from build123d import *

# Parameters (mm, degrees)
SKETCH_1_W                       = 990
SKETCH_1_H                       = 2
SM_BASE_FLANGE_1_DEPTH           = 60
SM_EDGE_FLANGE_1_STRIP_W         = 9
SM_EDGE_FLANGE_1_STRIP_H         = 2
SM_EDGE_FLANGE_1_STRIP_CUT_DEPTH = 990
SM_EDGE_FLANGE_1_DEPTH           = 990
SM_EDGE_FLANGE_2_STRIP_W         = 9
SM_EDGE_FLANGE_2_STRIP_H         = 2
SM_EDGE_FLANGE_2_STRIP_CUT_DEPTH = 990
SM_EDGE_FLANGE_2_DEPTH           = 990
SM_EDGE_FLANGE_3_STRIP_W         = 9
SM_EDGE_FLANGE_3_STRIP_H         = 2
SM_EDGE_FLANGE_3_STRIP_CUT_DEPTH = 990
SM_EDGE_FLANGE_3_DEPTH           = 990
SM_EDGE_FLANGE_4_STRIP_W         = 9
SM_EDGE_FLANGE_4_STRIP_H         = 2
SM_EDGE_FLANGE_4_STRIP_CUT_DEPTH = 990
SM_EDGE_FLANGE_4_DEPTH           = 990
HOLE_WIZARD_19_0_19_1_D          = 19
HOLE_WIZARD_M4_1_D               = 4
PATTERN_LINEAR_1_COUNT           = 2
PATTERN_LINEAR_1_PITCH           = 764.04
CUT_EXTRUDE_1_DEPTH              = 2
PATTERN_LINEAR_2_COUNT           = 2
PATTERN_LINEAR_2_PITCH           = 20
PATTERN_LINEAR_2_COUNT_DIR2      = 2
PATTERN_LINEAR_2_PITCH_DIR2      = 35
CUT_EXTRUDE_4_DEPTH              = 2
MIRROR_1_COPY_1_DEPTH            = 2
MIRROR_1_COPY_2_DEPTH            = 2
MIRROR_1_COPY_3_DEPTH            = 2
CUT_EXTRUDE_2_DEPTH              = 2
PATTERN_LINEAR_3_COUNT           = 6
PATTERN_LINEAR_3_PITCH           = 116


# Sheet-metal steps are written as plain solids
with BuildPart() as part:
    # Sketch 1 → 基体-法兰1 (new body)
    with BuildSketch(Plane.XY):
        with Locations((0, -1)):
            Rectangle(SKETCH_1_W, SKETCH_1_H)
    extrude(amount=SM_BASE_FLANGE_1_DEPTH)

    # 边线-法兰1 strip (across the edge) → 边线-法兰1 strip cut (cut)
    with BuildSketch(Plane(origin=(-495, -2, 0), x_dir=(0, 0, 1), z_dir=(1, 0, 0))):
        with Locations((-2, -1)):
            Rectangle(SM_EDGE_FLANGE_1_STRIP_W, SM_EDGE_FLANGE_1_STRIP_H)
    extrude(amount=SM_EDGE_FLANGE_1_STRIP_CUT_DEPTH, mode=Mode.SUBTRACT)

    # 边线-法兰1 section (across the edge) → 边线-法兰1 (add)
    with BuildSketch(Plane(origin=(-495, -2, 0), x_dir=(0, 0, 1), z_dir=(1, 0, 0))):
        with BuildLine():
            Line((0, 0.5), (0, 15))
            Line((0, 15), (2, 15))
            Line((2, 15), (2, 0.5))
            ThreePointArc((2, 0.5), (2.146446609, 0.146446609), (2.5, 0))
            Line((2.5, 0), (2.5, -2))
            ThreePointArc((2.5, -2), (0.732233047, -1.267766953), (0, 0.5))
        make_face()
    extrude(amount=SM_EDGE_FLANGE_1_DEPTH)

    # 边线-法兰2 strip (across the edge) → 边线-法兰2 strip cut (cut)
    with BuildSketch(Plane(origin=(495, -2, 60), x_dir=(0, 0, -1), z_dir=(-1, 0, 0))):
        with Locations((-2, -1)):
            Rectangle(SM_EDGE_FLANGE_2_STRIP_W, SM_EDGE_FLANGE_2_STRIP_H)
    extrude(amount=SM_EDGE_FLANGE_2_STRIP_CUT_DEPTH, mode=Mode.SUBTRACT)

    # 边线-法兰2 section (across the edge) → 边线-法兰2 (add)
    with BuildSketch(Plane(origin=(495, -2, 60), x_dir=(0, 0, -1), z_dir=(-1, 0, 0))):
        with BuildLine():
            Line((0, 0.5), (0, 15))
            Line((0, 15), (2, 15))
            Line((2, 15), (2, 0.5))
            ThreePointArc((2, 0.5), (2.146446609, 0.146446609), (2.5, 0))
            Line((2.5, 0), (2.5, -2))
            ThreePointArc((2.5, -2), (0.732233047, -1.267766953), (0, 0.5))
        make_face()
    extrude(amount=SM_EDGE_FLANGE_2_DEPTH)

    # 边线-法兰3 strip (across the edge) → 边线-法兰3 strip cut (cut)
    with BuildSketch(Plane(origin=(495, -17, 58), x_dir=(0, 1, 0), z_dir=(-1, 0, 0))):
        with Locations((-4, -1)):
            Rectangle(SM_EDGE_FLANGE_3_STRIP_W, SM_EDGE_FLANGE_3_STRIP_H)
    extrude(amount=SM_EDGE_FLANGE_3_STRIP_CUT_DEPTH, mode=Mode.SUBTRACT)

    # 边线-法兰3 section (across the edge) → 边线-法兰3 (add)
    with BuildSketch(Plane(origin=(495, -17, 58), x_dir=(0, 1, 0), z_dir=(-1, 0, 0))):
        with BuildLine():
            Line((-2, 0.5), (-2, 8))
            Line((-2, 8), (0, 8))
            Line((0, 8), (0, 0.5))
            ThreePointArc((0, 0.5), (0.146446609, 0.146446609), (0.5, 0))
            Line((0.5, 0), (0.5, -2))
            ThreePointArc((0.5, -2), (-1.267766953, -1.267766953), (-2, 0.5))
        make_face()
    extrude(amount=SM_EDGE_FLANGE_3_DEPTH)

    # 边线-法兰4 strip (across the edge) → 边线-法兰4 strip cut (cut)
    with BuildSketch(Plane(origin=(-495, -17, 2), x_dir=(0, 1, 0), z_dir=(1, 0, 0))):
        with Locations((-4, -1)):
            Rectangle(SM_EDGE_FLANGE_4_STRIP_W, SM_EDGE_FLANGE_4_STRIP_H)
    extrude(amount=SM_EDGE_FLANGE_4_STRIP_CUT_DEPTH, mode=Mode.SUBTRACT)

    # 边线-法兰4 section (across the edge) → 边线-法兰4 (add)
    with BuildSketch(Plane(origin=(-495, -17, 2), x_dir=(0, 1, 0), z_dir=(1, 0, 0))):
        with BuildLine():
            Line((-2, 0.5), (-2, 8))
            Line((-2, 8), (0, 8))
            Line((0, 8), (0, 0.5))
            ThreePointArc((0, 0.5), (0.146446609, 0.146446609), (0.5, 0))
            Line((0.5, 0), (0.5, -2))
            ThreePointArc((0.5, -2), (-1.267766953, -1.267766953), (-2, 0.5))
        make_face()
    extrude(amount=SM_EDGE_FLANGE_4_DEPTH)

    # Ø19.0 (19) 直径孔1 (through all)
    with Locations(Plane.XZ.offset(2)):
        with Locations((-382.02, 30), (382.02, 30)):
            Hole(HOLE_WIZARD_19_0_19_1_D / 2)

    # M4 螺纹孔1 (through all)
    with Locations(Plane.XZ.offset(2)):
        with Locations((-396.02, 30), (-368.02, 30), (-382.02, 44), (-382.02, 16)):
            hole_wizard_m4_1 = Hole(HOLE_WIZARD_M4_1_D / 2)

    # 阵列(线性)1: M4 螺纹孔1 ×2
    with Locations(*[(i * PATTERN_LINEAR_1_PITCH, 0, 0) for i in range(1, PATTERN_LINEAR_1_COUNT)]):
        add(hole_wizard_m4_1, mode=Mode.SUBTRACT)

    # 草图19 → 切除-拉伸1 (cut)
    with BuildSketch(Plane(origin=(0, 0, 0), x_dir=(1, 0, 0), z_dir=(0, 1, 0))):
        with BuildLine():
            Line((460.249565443, -15.5), (460.249565443, -9.5))
            ThreePointArc((460.249565443, -9.5), (462.999565443, -6.75), (465.749565443, -9.5))
            Line((465.749565443, -9.5), (465.749565443, -15.5))
            ThreePointArc((465.749565443, -15.5), (462.999565443, -18.25), (460.249565443, -15.5))
        make_face()
    cut_extrude_1 = extrude(amount=-CUT_EXTRUDE_1_DEPTH, mode=Mode.SUBTRACT)

    # 阵列(线性)2: Cut-Extrude 1 2 × 2
    with Locations(*[(i * PATTERN_LINEAR_2_PITCH, 0, j * PATTERN_LINEAR_2_PITCH_DIR2) for i in range(PATTERN_LINEAR_2_COUNT) for j in range(PATTERN_LINEAR_2_COUNT_DIR2) if (i, j) != (0, 0)]):
        add(cut_extrude_1, mode=Mode.SUBTRACT)

    # 草图23 → 切除-拉伸4 (cut)
    with BuildSketch(Plane.XZ.offset(19)):
        with BuildLine():
            Line((466.999565443, 10), (458.999565443, 10))
            ThreePointArc((458.999565443, 10), (462.999565443, 6), (466.999565443, 10))
        make_face()
        with BuildLine():
            Line((486.999565443, 10), (478.999565443, 10))
            ThreePointArc((478.999565443, 10), (482.999565443, 6), (486.999565443, 10))
        make_face()
        with BuildLine():
            Line((486.999565443, 50), (478.999565443, 50))
            ThreePointArc((478.999565443, 50), (482.999565443, 54), (486.999565443, 50))
        make_face()
        with BuildLine():
            Line((466.999565443, 50), (458.999565443, 50))
            ThreePointArc((458.999565443, 50), (462.999565443, 54), (466.999565443, 50))
        make_face()
    cut_extrude_4 = extrude(amount=-CUT_EXTRUDE_4_DEPTH, mode=Mode.SUBTRACT)

    # 镜向1: 切除-拉伸1, 切除-拉伸4 across plane
    add(cut_extrude_1.mirror(Plane(origin=(0, 0, 0), x_dir=(0, 0, 1), z_dir=(1, 0, 0))), mode=Mode.SUBTRACT)
    add(cut_extrude_4.mirror(Plane(origin=(0, 0, 0), x_dir=(0, 0, 1), z_dir=(1, 0, 0))), mode=Mode.SUBTRACT)

    # 镜向1 copy 1 sketch → 镜向1 copy 1 (cut)
    with BuildSketch(Plane(origin=(0, 0, 35), x_dir=(-1, 0, 0), z_dir=(0, 1, 0))):
        with BuildLine():
            Line((460.249565443, 15.5), (460.249565443, 9.5))
            ThreePointArc((460.249565443, 9.5), (462.999565443, 6.75), (465.749565443, 9.5))
            Line((465.749565443, 9.5), (465.749565443, 15.5))
            ThreePointArc((465.749565443, 15.5), (462.999565443, 18.25), (460.249565443, 15.5))
        make_face()
    extrude(amount=-MIRROR_1_COPY_1_DEPTH, mode=Mode.SUBTRACT)

    # 镜向1 copy 2 sketch → 镜向1 copy 2 (cut)
    with BuildSketch(Plane(origin=(-20, 0, 0), x_dir=(-1, 0, 0), z_dir=(0, 1, 0))):
        with BuildLine():
            Line((460.249565443, 15.5), (460.249565443, 9.5))
            ThreePointArc((460.249565443, 9.5), (462.999565443, 6.75), (465.749565443, 9.5))
            Line((465.749565443, 9.5), (465.749565443, 15.5))
            ThreePointArc((465.749565443, 15.5), (462.999565443, 18.25), (460.249565443, 15.5))
        make_face()
    extrude(amount=-MIRROR_1_COPY_2_DEPTH, mode=Mode.SUBTRACT)

    # 镜向1 copy 3 sketch → 镜向1 copy 3 (cut)
    with BuildSketch(Plane(origin=(-20, 0, 35), x_dir=(-1, 0, 0), z_dir=(0, 1, 0))):
        with BuildLine():
            Line((460.249565443, 15.5), (460.249565443, 9.5))
            ThreePointArc((460.249565443, 9.5), (462.999565443, 6.75), (465.749565443, 9.5))
            Line((465.749565443, 9.5), (465.749565443, 15.5))
            ThreePointArc((465.749565443, 15.5), (462.999565443, 18.25), (460.249565443, 15.5))
        make_face()
    extrude(amount=-MIRROR_1_COPY_3_DEPTH, mode=Mode.SUBTRACT)

    # 草图20 → 切除-拉伸2 (cut)
    with BuildSketch(Plane(origin=(0, 0, 0), x_dir=(1, 0, 0), z_dir=(0, 1, 0))):
        with BuildLine():
            Line((-335, -10), (-245, -10))
            ThreePointArc((-245, -10), (-241.464466094, -11.464466094), (-240, -15))
            Line((-240, -15), (-240, -45))
            ThreePointArc((-240, -45), (-241.464466094, -48.535533906), (-245, -50))
            Line((-245, -50), (-335, -50))
            ThreePointArc((-335, -50), (-338.535533906, -48.535533906), (-340, -45))
            Line((-340, -45), (-340, -15))
            ThreePointArc((-340, -15), (-338.535533906, -11.464466094), (-335, -10))
        make_face()
    cut_extrude_2 = extrude(amount=-CUT_EXTRUDE_2_DEPTH, mode=Mode.SUBTRACT)

    # 阵列(线性)3: 切除-拉伸2 ×6
    with Locations(*[(i * PATTERN_LINEAR_3_PITCH, 0, 0) for i in range(1, PATTERN_LINEAR_3_COUNT)]):
        add(cut_extrude_2, mode=Mode.SUBTRACT)


solid = part.part
The model under review builds one solid part; all positions refer to its coordinate system, in mm. A direction names the side the tool comes from. Give positions to 0.01 mm unless a question says otherwise; leave off trailing zeros. Order: outer loops, then holes, each group sorted by start corner. A loop starts at its lowest first (then second) coordinate and runs counter-clockwise, first axis right, second up. Notation, with made-up numbers: M -37.5,22 L -0.5,22 A14 ccw -0.5,33 Z; hole C 30.5,-19.5 d1. An arc over 180 degrees is marked long. Answer in a Markdown table with one row per item. Add a question column.
1. Add section B-B on x = 433.5. State the section outline as (y, z) points, plus the area to 3 significant figures.
2. Machinability: for faces 3 (the flat face through (-7, -2, 30)), 4 (the flat face through (-7, 0, 30)), which of the approach directions +Z, -Z, +X, -X, +Y, -Y give a long, thin tool a straight path to every point of the face, cutting with its end or side? Answer none if there is none.
3. Add section A-A on y = -11.5. State the section outline as (x, z) points.
4. For pin 1 Ø0.6 at (x, y) = (161, -1) entering from -Z; pin 2 Ø3 at (x, z) = (362, 42) entering from -Y; pin 3 Ø1 at (x, y) = (-54, -1) entering from +Z, all flat-tipped, find the tip position at first contact; note any pin that passes through.
5. Mouldability with a two-part tool opening along Z and no side actions: class faces 1 (the flat face through (-495, -1.7, 30.1)), 2 (the cylindrical face through (-372.53, -0.99, 30.42)) as released by +Z, released by -Z, zero draft, split by the parting line, or undercut.
6. To check wall thickness, follow line 1 along Z through (x, y) = (-280.5, -3.75); line 2 along Y through (x, z) = (350.5, 5); line 3 along Z through (x, y) = (368.02, -1). State the ranges of each line that lie inside material, in increasing order.
The answers:
| question | item | result |
|---|---|---|
| 1 | outline | M -19,2.5 A2.5 ccw -16.5,0 L -2.5,0 A2.5 ccw 0,2.5 L 0,57.5 A2.5 ccw -2.5,60 L -16.5,60 A2.5 ccw -19,57.5 L -19,50 L -17,50 L -17,57.5 A0.5 cw -16.5,58 L -2.5,58 A0.5 cw -2,57.5 L -2,2.5 A0.5 cw -2.5,2 L -16.5,2 A0.5 cw -17,2.5 L -17,10 L -19,10 Z |
| 1 | area | 215 mm2 |
| 2 | face 3 | +X, -X |
| 2 | face 4 | +Z, -Z, +X, -X, +Y |
| 3 | outline | M -495,0 L 495,0 L 495,2 L -495,2 Z; M -495,58 L 495,58 L 495,60 L -495,60 Z |
| 4 | pin 1 | z = 0.31 |
| 4 | pin 2 | y = -2 |
| 4 | pin 3 | z = 59.79 |
| 5 | face 1 | zero draft |
| 5 | face 2 | undercut |
| 6 | line 1 | 0 to 2, 58 to 60 |
| 6 | line 2 | -19 to -17, -2 to 0 |
| 6 | line 3 | 0.5 to 28, 32 to 59.5 |
